Input: part model. Units: mm. Frame: model coordinates. Face numbers are marked on the shaded views. A direction names the side the tool comes from. Give positions to 0.01 mm unless a question says otherwise; leave off trailing zeros. Write each loop counter-clockwise with the first axis right and the second up, starting at its lowest first coordinate (ties: lowest second). Pieces come first, ordered by that corner, then holes.
```python
from build123d import *

# Parameters (mm, degrees)
F0_W      = 12
F0_H      = 25
F1_DEPTH  = 8
F2_SIZE   = 2
F3_SIZE   = 2
F4_R      = 2.25
F5_DEPTH  = 25
F6_R      = 4
F7_DEPTH  = 7
F8_R      = 4
F9_DEPTH  = 25
F10_W     = 8
F10_H     = 27.262656
F11_DEPTH = 1


with BuildPart() as f1:
    # F0 (on Front) → F1 (new body)
    with BuildSketch(Plane.XZ):
        with Locations((1.81407, 3.270565)):
            Rectangle(F0_W, F0_H)
    extrude(amount=F1_DEPTH)

    # F2
    f2_edges = [f1.edges().sort_by_distance(p)[0] for p in [
        (-4.18593, -4, 15.770565),
    ]]
    chamfer(f2_edges, length=F2_SIZE)

    # F3
    f3_edges = [f1.edges().sort_by_distance(p)[0] for p in [
        (7.81407, -4, 15.770565),
        (7.81407, -4, -9.229435),
        (-4.18593, -4, -9.229435),
    ]]
    chamfer(f3_edges, length=F3_SIZE)

    # F4 (on face) → F5 (cut)
    with BuildSketch(Plane.XZ.offset(8)):
        with Locations((1.81407, -4.979435)):
            Circle(F4_R)
        with Locations((1.81407, 11.520565)):
            Circle(F4_R)
    extrude(amount=-F5_DEPTH, mode=Mode.SUBTRACT)

    # F6 (on face) → F7 (cut)
    with BuildSketch(Plane.XZ.offset(8)):
        with Locations((1.81407, 11.520565)):
            Circle(F6_R)
        with Locations((1.81407, -4.979435)):
            Circle(F6_R)
    extrude(amount=-F7_DEPTH, mode=Mode.SUBTRACT)

    # F8 (on Front) → F9 (cut)
    with BuildSketch(Plane.XZ):
        with Locations((1.887019, 3.270565)):
            Circle(F8_R)
    extrude(amount=F9_DEPTH, mode=Mode.SUBTRACT)

    # F10 (on face) → F11 (cut)
    with BuildSketch(Plane(origin=(-4.18593, 0, 0), x_dir=(0, -1, 0), z_dir=(-1, 0, 0))):
        with Locations((4, 2.890538)):
            Rectangle(F10_W, F10_H)
    extrude(amount=-F11_DEPTH, mode=Mode.SUBTRACT)


solid = f1.part
```
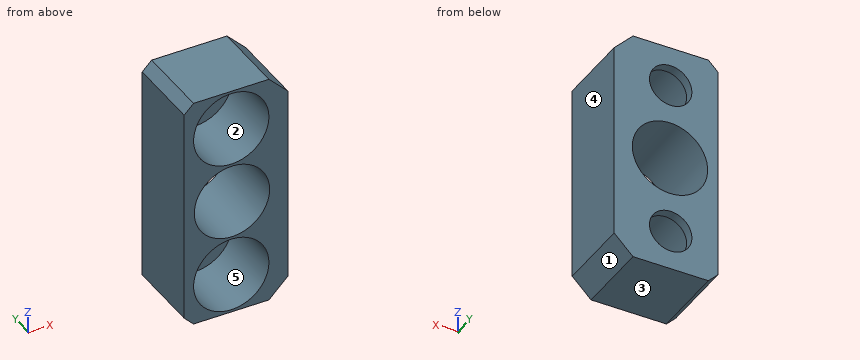
Q1. Section B-B, the plane x = -1.75. Return the cut outline in (y, z), then the cut area to 3 significant figures.
Q2. Mould query, pull axis Z, two halves, no side actions, for the marked faces 3, 4 and 5. Classes: +Z half, -Z half, draft (parallel to the pull), parting line (faces both ways), or undercut.
Q3. Access query for the marked faces 1 and 2. Directions: +Z, -Z, +X, -X, +Y, -Y. A direction counts if a zero-diameter tool reaches every point of the face in a straight line with its end or side. Return the directions, or none.
Q4. Material intervals for line 1 along Z through (x, y) = (2, -6.5); line 2 along Z through (x, y) = (3.75, -4.5); line 3 along Y through (x, z) = (-0.75, 11.75), sorted ascending.
Q5. Section C-C, the plane y = -4. Return the cut outline in (x, z), then the cut area to 3 significant figures.
Q6. Section D-D, the plane z = 7. Return the cut outline in (x, y), then the cut area to 3 significant figures.
Q7. Pin query (flat end, axial travel): pin 1 (5 mm diameter, centred on x = 1.81, z = 11.52, fed in from -Y). Return the tip coordinate at first contact, or that it passes through.
Q8. Section A-A, the plane z = -3. Return the cut outline in (x, y).
Solutions:
1. outline: (-8, -9.23) - (0, -9.23) - (0, 1.61) - (-8, 1.61) - (-8, -3.16) - (-1, -3.16) - (-1, -6.8) - (-8, -6.8) - close; (-8, 4.94) - (0, 4.94) - (0, 15.77) - (-8, 15.77) - (-8, 13.34) - (-1, 13.34) - (-1, 9.7) - (-8, 9.7) - close
1. area: 123 mm2
2. face 3: -Z half
2. face 4: draft
2. face 5: undercut
3. face 1: -Z, +X, +Y, -Y
3. face 2: -Y
4. line 1: z = -9.23 to -8.98, -0.98 to -0.73, 7.27 to 7.52, 15.52 to 15.77
4. line 2: z = -9.23 to -8.48, -1.48 to -0.27, 6.81 to 8.02, 15.02 to 15.77
4. line 3: y = -1 to 0
5. outline: (-3.19, -8.23) - (-2.19, -9.23) - (5.81, -9.23) - (7.81, -7.23) - (7.81, 13.77) - (5.81, 15.77) - (-2.19, 15.77) - (-3.19, 14.77) - close; hole circle Ø8 at (1.81, -4.98); hole circle Ø8 at (1.81, 11.52); hole circle Ø8 at (1.89, 3.27)
5. area: 119 mm2
6. outline: (-3.19, -8) - (0.44, -8) - (0.44, 0) - (-3.19, 0) - close; (3.33, -8) - (7.81, -8) - (7.81, 0) - (3.33, 0) - close
6. area: 64.9 mm2
7. pin 1: stops at y = -1
8. outline: (-3.19, -8) - (-1.66, -8) - (-1.66, -1) - (0.74, -1) - (0.74, 0) - (-3.19, 0) - close; (2.88, -1) - (5.29, -1) - (5.29, -8) - (7.81, -8) - (7.81, 0) - (2.88, 0) - close
